from build123d import *

# Parameters (mm, degrees)
F2_T = -2.54


# Not quite as in the source:
# - a fillet or chamfer that OpenCascade refuses, or shapes differently, is made with other operations: its cross-section is extruded or revolved along the edge and cut away or added
# - the program builds the solid bodies; features that only make, move or delete a surface that nothing else refers to are left out


with BuildPart() as f1:
    # F0 (on Front) → F1 (revolve)
    with BuildSketch(Plane.XZ):
        Polygon((39.6217921842, 43.7875076047), (-5.3782078158, 43.7875076047), (-5.3782078158, -56.2124923953), (29.6217921842, -56.2124923953), (30.6275011268, -46.1554029698), (38.3154473181, 30.724058944), align=None)
    revolve(axis=Axis((-5.3782078158, 0, -6.2124923953), (0, 0, -1)))

    # F2
    f2_openings = [f1.faces().sort_by_distance(p)[0] for p in [
        (-5.378208, 0, 43.787508),
    ]]
    offset(amount=F2_T, openings=f2_openings, kind=Kind.INTERSECTION)

    # F3: fillet of radius 5.08 on 3 edges, made by hand

    # F3_s1 → F3_t2 (revolve, cut)
    with BuildSketch(Plane.XZ):
        with BuildLine():
            ThreePointArc((30.079244295, -51.6379712879), (28.4331623981, -54.8990712658), (25.0244553687, -56.2124923953))
            Line((25.0244553687, -56.2124923953), (29.6217921842, -56.2124923953))
            Line((29.6217921842, -56.2124923953), (30.079244295, -51.6379712879))
        make_face()
    revolve(axis=Axis((-5.3782078158, 0, -56.2124923953), (0, 0, -1)), mode=Mode.SUBTRACT)

    # F3_s3 → F3_t4 (revolve, cut)
    with BuildSketch(Plane.XZ):
        with BuildLine():
            ThreePointArc((39.1587606775, 39.1571925375), (38.7342868185, 41.7523083311), (37.0691237764, 43.7875076047))
            Line((37.0691237764, 43.7875076047), (39.6217921842, 43.7875076047))
            Line((39.6217921842, 43.7875076047), (39.1587606775, 39.1571925375))
        make_face()
    revolve(axis=Axis((-5.3782078158, 0, 43.7875076047), (0, 0, -1)), mode=Mode.SUBTRACT)


solid = f1.part
Design review of the part built by this model. Coordinates are the model's own, in mm. Round coordinates to 2 decimals unless told otherwise and drop trailing zeros. Order: outer loops, then holes, each group sorted by start corner. A loop starts at its lowest first (then second) coordinate and runs counter-clockwise, first axis right, second up.
1) Consider section A-A (z = 37). State the section outline as (x, y) points.
The answers:
outline: circle Ø88.64 at (-5.38, 0); hole circle Ø83.54 at (-5.38, 0)
2) Consider section B-B (z = -1.5). State the section outline as (x, y) points.
The answers:
outline: circle Ø80.94 at (-5.38, 0); hole circle Ø75.84 at (-5.38, 0)
3) For L1, parallel to Z at x = 15.5, y = -5.5; L2, parallel to Y at x = -9.5, z = 20.5; L3, parallel to X at y = -30, z = 33.5, list the stretches that pass through material, from the lowest coordinate up.
The answers:
L1: z = -56.21 to -53.67
L2: y = -42.47 to -39.91, 39.91 to 42.47
L3: x = -37.53 to -33.94, 23.18 to 26.77
4) Draft analysis for pull direction Y (two halves, no side actions). For faces 1 (the flat face through (-5, 0, -53.672)), 2 (the flat face through (-5, 0, -56.212)), state which applies: released by +Y, released by -Y, zero draft, split by the parting line, or undercut.
The answers:
face 1: undercut
face 2: zero draft
5) Clearance check with flat-ended pins moving along their axes: pin 1 Ø12 at (x, z) = (-14, -11.5) entering from -Y; pin 2 Ø8 at (x, z) = (-39, 23.5) entering from +Y; pin 3 Ø8 at (y, z) = (15, -22.5) entering from -X. State where each tip first meets the part, or that it passes through.
The answers:
pin 1: stops at y = -39.66
pin 2: stops at y = 31.17
pin 3: stops at x = -42.21
